Could you check a few things on this drawing? It's one solid part, dimensions in mm from its lowest x, y, z. Give positions to 0.01 mm unless a question says otherwise; leave off trailing zeros. Loops run counter-clockwise (first coordinate to the right, second up) from the corner with the lowest first, then second, coordinate; pieces in that order, holes last. Notation, with made-up numbers: (-31.75, 9.25) - (-3.75, 9.25) arc R19 ccw to (-3.75, 31.25) - close; hole circle Ø7 at (3, 36.25). An arc over 180 degrees is marked (long way). One line per item, written item: value. Start each with the question number.
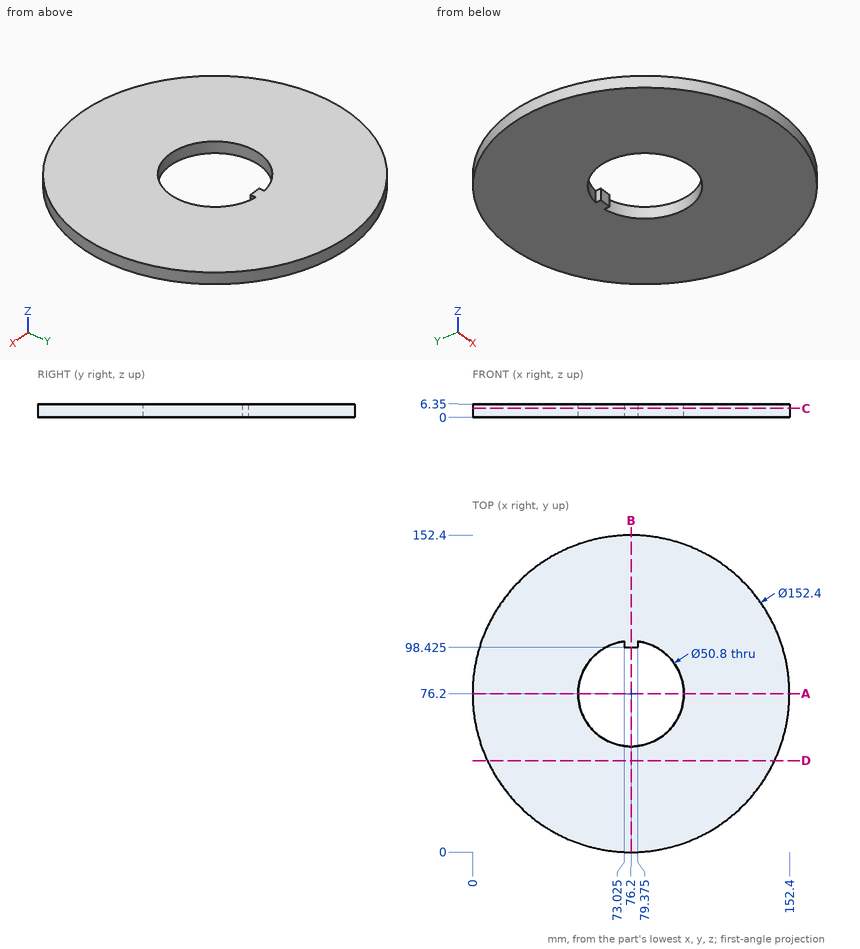
(1) If we section it at A-A on y = 76.2: List the corners of the cut face in (x, z) for me, plus the area to 3 significant figures.
(2) If we section it at C-C on z = 4.25: List the corners of the cut face in (x, y) for me (3 decimals).
(3) If we section it at B-B on x = 76.2: List the corners of the cut face in (y, z) for me (3 decimals), plus the area to 3 significant figures.
(4) Will these pins go through, and if not, where does the flat tip stop? pin 1 (4 mm diameter, centred on x = 95, y = 88.5, fed in from +Z); pin 2 (3 mm diameter, centred on x = 46.5, y = 91.5, fed in from -Z); pin 3 (1 mm diameter, centred on x = 51.5, z = 3, fed in from -Y); pin 4 (0.9 mm diameter, centred on y = 100, z = 3, fed in from -X).
(5) If we section it at D-D on y = 44: List the corners of the cut face in (x, z) for me.
(6) Please list where these lines run through material, in increasing order: probe 1 along Y at (x, z) = (76.2, 2.25) (3 decimals); probe 2 along X at (y, z) = (79.5, 5); probe 3 along X at (y, z) = (97.5, 4.75). Write a range as from..to.
Found:
1. outline: (0, 0) - (50.8, 0) - (50.8, 6.35) - (0, 6.35) - close; (101.6, 0) - (152.4, 0) - (152.4, 6.35) - (101.6, 6.35) - close
1. area: 645 mm^2
2. outline: circle Ø152.4 at (76.2, 76.2); hole (73.025, 98.425) - (73.025, 101.401) arc R25.4 ccw (long way) to (79.375, 101.401) - (79.375, 98.425) - close
3. outline: (0, 0) - (50.8, 0) - (50.8, 6.35) - (0, 6.35) - close; (98.425, 0) - (152.4, 0) - (152.4, 6.35) - (98.425, 6.35) - close
3. area: 665 mm^2
4. pin 1: through
4. pin 2: z = 0
4. pin 3: y = 3.94
4. pin 4: x = 3.67
5. outline: (7.14, 0) - (145.26, 0) - (145.26, 6.35) - (7.14, 6.35) - close
6. probe 1: 0..50.8, 98.425..152.4
6. probe 2: 0.07..51.02, 101.38..152.33
6. probe 3: 3.04..62.36, 90.04..149.36
